```python
from build123d import *

# Parameters (mm, degrees)
F0_W     = 167.259
F0_H     = 133.858
F0_R     = 6.604
F0_R_2   = 3.429
F0_R_3   = 8.255
F1_DEPTH = 12.7
F2_W     = 167.259
F2_H     = 133.858
F3_DEPTH = 6.35
F4_R     = 12.7


with BuildPart() as f1:
    # F0 (on Top) → F1 (new body)
    with BuildSketch(Plane.XY):
        with Locations((26.2255, 0)):
            Rectangle(F0_W, F0_H)
        with Locations((-38.1, -38.1)):
            Circle(F0_R, mode=Mode.SUBTRACT)
        with Locations((0, -50.8)):
            Circle(F0_R_2, mode=Mode.SUBTRACT)
        with Locations((25.4, -50.8)):
            Circle(F0_R_2, mode=Mode.SUBTRACT)
        with BuildLine():
            ThreePointArc((3.429, -25.4), (-2.424669, -27.824669), (0, -21.971))
            ThreePointArc((0, -21.971), (2.424669, -22.975331), (3.429, -25.4))
        make_face(mode=Mode.SUBTRACT)
        with Locations((25.4, -25.4)):
            Circle(F0_R_2, mode=Mode.SUBTRACT)
        with Locations((50.8, -50.8)):
            Circle(F0_R_2, mode=Mode.SUBTRACT)
        with Locations((88.9, -38.1)):
            Circle(F0_R_3, mode=Mode.SUBTRACT)
        with Locations((50.8, -25.4)):
            Circle(F0_R_2, mode=Mode.SUBTRACT)
        with Locations((-38.1, 0)):
            Circle(F0_R, mode=Mode.SUBTRACT)
        with BuildLine():
            ThreePointArc((0, -3.429), (-2.424669, 2.424669), (3.429, 0))
            ThreePointArc((3.429, 0), (2.424669, -2.424669), (0, -3.429))
        make_face(mode=Mode.SUBTRACT)
        with BuildLine():
            ThreePointArc((28.829, 0), (25.4, -3.429), (21.971, 0))
            ThreePointArc((21.971, 0), (25.4, 3.429), (28.829, 0))
        make_face(mode=Mode.SUBTRACT)
        with Locations((0, 25.4)):
            Circle(F0_R_2, mode=Mode.SUBTRACT)
        with Locations((25.4, 25.4)):
            Circle(F0_R_2, mode=Mode.SUBTRACT)
        with Locations((-38.1, 38.1)):
            Circle(F0_R, mode=Mode.SUBTRACT)
        with Locations((0, 50.8)):
            Circle(F0_R_2, mode=Mode.SUBTRACT)
        with Locations((25.4, 50.8)):
            Circle(F0_R_2, mode=Mode.SUBTRACT)
        with Locations((50.8, 0)):
            Circle(F0_R_2, mode=Mode.SUBTRACT)
        with Locations((50.8, 25.4)):
            Circle(F0_R_2, mode=Mode.SUBTRACT)
        with Locations((88.9, 0)):
            Circle(F0_R_3, mode=Mode.SUBTRACT)
        with Locations((50.8, 50.8)):
            Circle(F0_R_2, mode=Mode.SUBTRACT)
        with Locations((88.9, 38.1)):
            Circle(F0_R_3, mode=Mode.SUBTRACT)
    extrude(amount=F1_DEPTH)

    # F2 (on face) → F3 (join)
    with BuildSketch(Plane(origin=(0, 0, 0), x_dir=(1, 0, 0), z_dir=(0, 0, -1))):
        with Locations((26.2255, 0)):
            Rectangle(F2_W, F2_H)
    extrude(amount=F3_DEPTH)

    # F4
    f4_edges = [f1.edges().sort_by_distance(p)[0] for p in [
        (-57.404, -66.929, 3.175),
        (-57.404, 66.929, 3.175),
        (109.855, -66.929, 3.175),
        (109.855, 66.929, 3.175),
    ]]
    fillet(f4_edges, radius=F4_R)


solid = f1.part
```
The model under review builds one solid part; all positions refer to its coordinate system, in mm. A direction names the side the tool comes from. Give positions to 0.01 mm unless a question says otherwise; leave off trailing zeros. Write each loop counter-clockwise with the first axis right and the second up, starting at its lowest first coordinate (ties: lowest second). Pieces come first, ordered by that corner, then holes. Notation, with made-up numbers: M -5.5,44 L 7.5,44 A22 cw 7.5,57 Z; hole C -10,72.25 d6. An arc over 180 degrees is marked long. Write each question's results on one line, items separated by ' | '. Start each with the question number.
1. Insertion check: pin 1 Ø3.5 at (x, y) = (26.5, -24.5) entering from +Z; pin 2 Ø5.5 at (x, y) = (26.5, 49.5) entering from +Z. Each pin has a flat end and moves straight along its axis. Give the tip position at first contact, or say it passes through.
2. For faces 4 (the flat face through (0, 0, 0)), 5 (the cylindrical face through (106.233, -63.11, 3.308)), list the 3-axis set-ups (+Z, -Z, +X, -X, +Y, -Y) from which the entire face can be reached by the end or side of a thin tool; tool diameter is ignored.
3. We need section D-D (x = 25.4). Write out the cut boundary in (y, z).
4. We need section A-A (x = -38.1). Write out the cut boundary in (y, z).
5. We need section C-C (z = 4.5). Count the separate pieces of the cut face and the enclosed holes in it, and give its area (3 significant figures).
6. Mouldability with a two-part tool opening along X and no side actions: class faces 1 (the cylindrical face through (82.349, -43.123, 6.261)), 2 (the flat face through (109.855, 1, 3)), 3 (the flat face through (89, 38, 0)) as released by +X, released by -X, zero draft, split by the parting line, or undercut.
7. For probe 1 along Y at (x, z) = (50.8, 6.25); probe 2 along X at (y, z) = (44, 3.5) (3 decimals); probe 3 along X at (y, z) = (-26, 9.5) (3 decimals), list the stretches that pass through material, from the lowest coordinate up. Write a range as [from, to].
8. We need section B-B (y = 50.8). Write out the cut boundary in (x, z) (3 decimals).
Results found:
1) pin 1: stops at z = 0 | pin 2: stops at z = 12.7
2) face 4: +Z | face 5: +Z, -Z, +X, -Y
3) outline: M -66.93,-6.35 L 66.93,-6.35 L 66.93,12.7 L 54.23,12.7 L 54.23,0 L 47.37,0 L 47.37,12.7 L 28.83,12.7 L 28.83,0 L 21.97,0 L 21.97,12.7 L 3.43,12.7 L 3.43,0 L -3.43,0 L -3.43,12.7 L -21.97,12.7 L -21.97,0 L -28.83,0 L -28.83,12.7 L -47.37,12.7 L -47.37,0 L -54.23,0 L -54.23,12.7 L -66.93,12.7 Z
4) outline: M -66.93,-6.35 L 66.93,-6.35 L 66.93,12.7 L 44.7,12.7 L 44.7,0 L 31.5,0 L 31.5,12.7 L 6.6,12.7 L 6.6,0 L -6.6,0 L -6.6,12.7 L -31.5,12.7 L -31.5,0 L -44.7,0 L -44.7,12.7 L -66.93,12.7 Z
5) separate pieces: 1 | enclosed holes: 21 | area: 20,600 mm^2
6) face 1: undercut | face 2: released by +X | face 3: undercut
7) probe 1: y = [-66.93, -54.23], [-47.37, -28.83], [-21.97, -3.43], [3.43, 21.97], [28.83, 47.37], [54.23, 66.93] | probe 2: x = [-57.404, -41.067], [-35.133, 83.126], [94.674, 109.855] | probe 3: x = [-57.404, -3.376], [3.376, 22.024], [28.776, 47.424], [54.176, 109.855]
8) outline: M -57.404,-6.35 L 109.855,-6.35 L 109.855,12.7 L 54.229,12.7 L 54.229,0 L 47.371,0 L 47.371,12.7 L 28.829,12.7 L 28.829,0 L 21.971,0 L 21.971,12.7 L 3.429,12.7 L 3.429,0 L -3.429,0 L -3.429,12.7 L -57.404,12.7 Z
